Verification items for this drawing (mm, ordinates from the low corner). A direction names the side the tool comes from. Coordinates: 2 decimals unless noted, no trailing zeros. Order: outer loops, then holes, each group sorted by start corner. A loop starts at its lowest first (then second) coordinate and runs counter-clockwise, first axis right, second up. Notation, with made-up numbers: M -24,77 L 9,77 A16 cw 9,87 Z; hole C 6,-9 d11. An arc over 180 degrees is marked long. Write item = value, one per line.
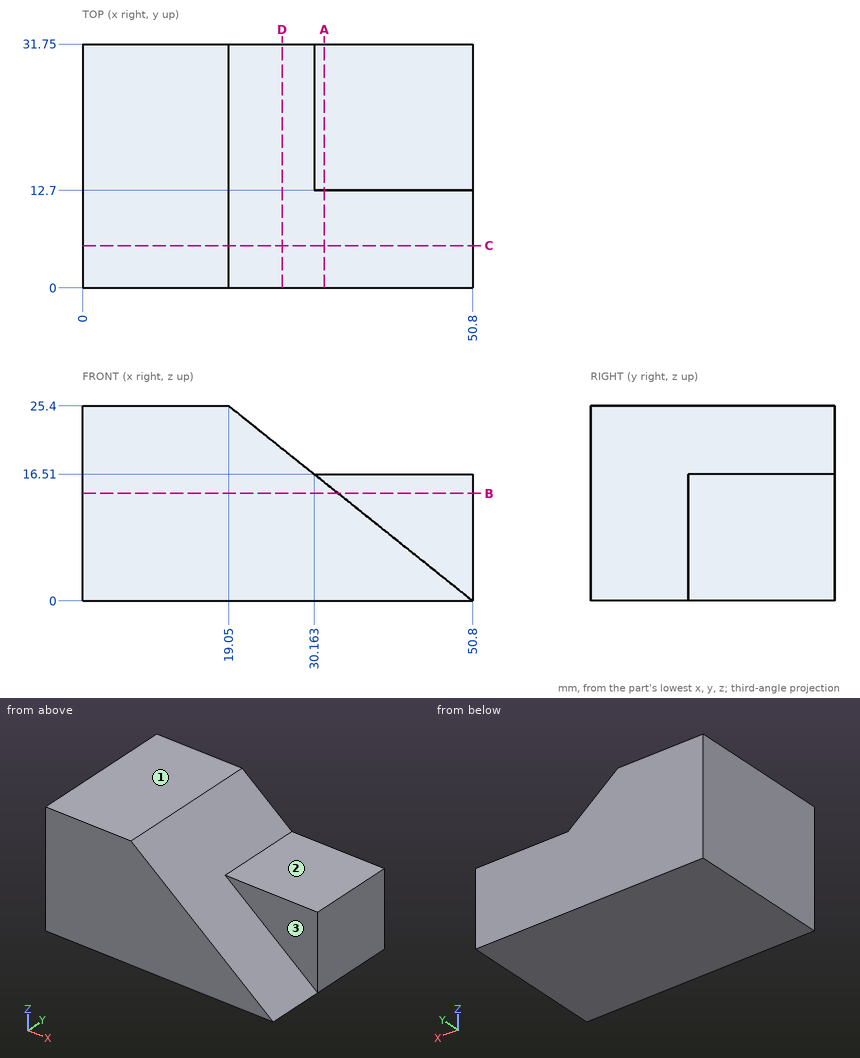
Item 1: Sectioned sample at D-D, the plane x = 26. Enter the section's corners in (y, z), then the cut area to 3 significant figures.
Report:
outline = M 0,0 L 31.75,0 L 31.75,19.84 L 0,19.84 Z
area = 630 mm^2
Item 2: Sectioned sample at C-C, the plane y = 5.5. Enter the section's corners in (x, z), then the cut area to 3 significant figures.
Report:
outline = M 0,0 L 50.8,0 L 19.05,25.4 L 0,25.4 Z
area = 887 mm^2
Item 3: Scan lines: L1, parallel to Z at x = 42, y = 14; L2, parallel to X at y = 1.5, z = 11.75 (1 decimal); L3, parallel to X at y = 5, z = 11. Record each from-to range of solid material in increasing order. Write a range as from..to.
Report:
L1 = 0..16.51
L2 = 0..36.1
L3 = 0..37.05
Item 4: Gauge pin test, flat ends, axial feed: pin 1 (4 mm diameter, centred on x = 27, y = 11.5, fed in from +Z); pin 2 (4 mm diameter, centred on y = 9, z = 5, fed in from +X); pin 3 (5.5 mm diameter, centred on x = 38.5, y = 19, fed in from +Z). Record the tip position at first contact, or that the pin passes through.
Report:
pin_1 = 20.64
pin_2 = 47.05
pin_3 = 16.51
Item 5: Sectioned sample at A-A, the plane x = 31.5. Enter the section's corners in (y, z), then the cut area to 3 significant figures.
Report:
outline = M 0,0 L 31.75,0 L 31.75,16.51 L 12.7,16.51 L 12.7,15.44 L 0,15.44 Z
area = 511 mm^2
Item 6: Sectioned sample at B-B, the plane z = 14. Enter the section's corners in (x, y), then the cut area to 3 significant figures.
Report:
outline = M 0,0 L 33.3,0 L 33.3,12.7 L 50.8,12.7 L 50.8,31.75 L 0,31.75 Z
area = 1,390 mm^2
Item 7: Tool access check on the marked faces 1, 2 and 3. Record the directions out of +Z, -Z, +X, -X, +Y, -Y that give a thin tool (end or side, any length) a straight path to the whole face; none if there is none.
Report:
face_1 = +Z, +X, -X, +Y, -Y
face_2 = +Z, +X, +Y, -Y
face_3 = +Z, +X, -Y
